Part print with two shaded views. Sizes in mm from the minimum x, y, z corner. Round coordinates to 2 decimals unless told otherwise and drop trailing zeros. Write each loop counter-clockwise with the first axis right and the second up, starting at its lowest first coordinate (ties: lowest second). Pieces come first, ordered by that corner, then holes. Notation, with made-up numbers: (46.5, 11.25) -> (55.5, 11.25) arc R19 cw to (55.5, 40.25) -> close; hole circle Ø7 at (27.25, 64). An arc over 180 degrees is marked (long way). Answer as CSV lines item,"result".
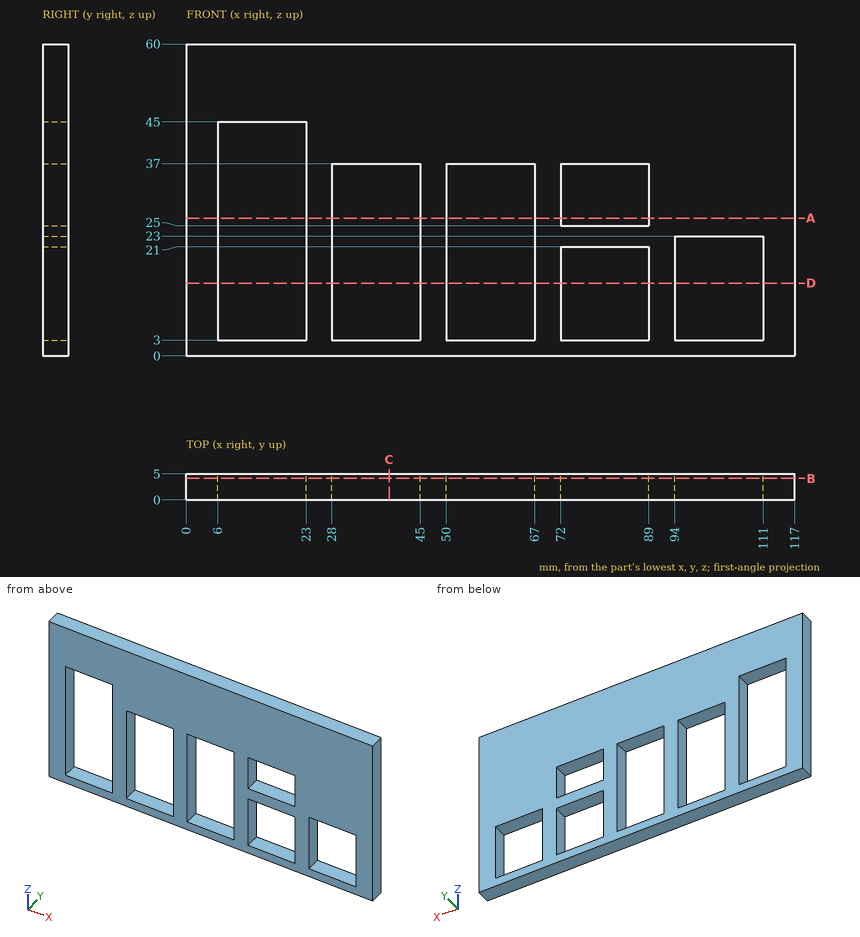
1. Cut at D-D, the plane z = 14. Write the cut outline in (x, y).
Results found:
outline,"(0, 0) -> (6, 0) -> (6, 5) -> (0, 5) -> close; (23, 0) -> (28, 0) -> (28, 5) -> (23, 5) -> close; (45, 0) -> (50, 0) -> (50, 5) -> (45, 5) -> close; (67, 0) -> (72, 0) -> (72, 5) -> (67, 5) -> close; (89, 0) -> (94, 0) -> (94, 5) -> (89, 5) -> close; (111, 0) -> (117, 0) -> (117, 5) -> (111, 5) -> close"
2. Cut at A-A, the plane z = 26.5. Write the cut outline in (x, y), then the cut area to 3 significant figures.
Results found:
outline,"(0, 0) -> (6, 0) -> (6, 5) -> (0, 5) -> close; (23, 0) -> (28, 0) -> (28, 5) -> (23, 5) -> close; (45, 0) -> (50, 0) -> (50, 5) -> (45, 5) -> close; (67, 0) -> (72, 0) -> (72, 5) -> (67, 5) -> close; (89, 0) -> (117, 0) -> (117, 5) -> (89, 5) -> close"
area,"245 mm2"
3. Probe line 1 along X through (y, z) = (4.75, 35); line 2 along X through (y, z) = (3.25, 13); line 3 along X through (y, z) = (4.7, 24). List the from-to ranges inside material, lowest first.
Results found:
line 1,"x = 0 to 6, 23 to 28, 45 to 50, 67 to 72, 89 to 117"
line 2,"x = 0 to 6, 23 to 28, 45 to 50, 67 to 72, 89 to 94, 111 to 117"
line 3,"x = 0 to 6, 23 to 28, 45 to 50, 67 to 117"
4. Cut at B-B, the plane y = 4.1. Write the cut outline in (x, z), then the cut area to 3 significant figures.
Results found:
outline,"(0, 0) -> (117, 0) -> (117, 60) -> (0, 60) -> close; hole (6, 3) -> (23, 3) -> (23, 45) -> (6, 45) -> close; hole (28, 3) -> (45, 3) -> (45, 37) -> (28, 37) -> close; hole (50, 3) -> (67, 3) -> (67, 37) -> (50, 37) -> close; hole (72, 3) -> (89, 3) -> (89, 21) -> (72, 21) -> close; hole (72, 25) -> (89, 25) -> (89, 37) -> (72, 37) -> close; hole (94, 3) -> (111, 3) -> (111, 23) -> (94, 23) -> close"
area,"4,300 mm2"
5. Cut at C-C, the plane x = 39. Write the cut outline in (y, z), then the cut area to 3 significant figures.
Results found:
outline,"(0, 0) -> (5, 0) -> (5, 3) -> (0, 3) -> close; (0, 37) -> (5, 37) -> (5, 60) -> (0, 60) -> close"
area,"130 mm2"
